```python
from build123d import *

# Parameters (mm, degrees)
SKETCH_1_R          = 3
SKETCH_1_R_2        = 5
EXTRUDE_1_DEPTH     = 4
CUT_EXTRUDE_1_DEPTH = 3


with BuildPart() as part:
    # 草图1 → 凸台-拉伸1 (new, symmetric)
    with BuildSketch(Plane(origin=(0, 0, 0), x_dir=(1, 0, 0), z_dir=(0, 1, 0))):
        with BuildLine():
            ThreePointArc((-0.330275229, 5.99090296), (-6, 0), (-0.330275229, -5.99090296))
            Line((-0.330275229, -5.99090296), (54.004587156, -8.98635444))
            ThreePointArc((54.004587156, -8.98635444), (63.5, 0), (54.004587156, 8.98635444))
            Line((54.004587156, 8.98635444), (-0.330275229, 5.99090296))
        make_face()
        with Locations(Location((0, 0, 0), (0, 0, 270))):
            Circle(SKETCH_1_R, mode=Mode.SUBTRACT)
        with Locations(Location((54.5, 0, 0), (0, 0, 270))):
            Circle(SKETCH_1_R_2, mode=Mode.SUBTRACT)
    extrude(amount=EXTRUDE_1_DEPTH, both=True)

    # 草图2 → 切除-拉伸1 (cut)
    with BuildSketch(Plane(origin=(0, 4, 0), x_dir=(1, 0, 0), z_dir=(0, 1, 0))):
        Polygon((26.837155963, 7.4886287), (11.750234203, -6.65689489), (-12.859516692, -6.65689489), (-12.859516692, 10.73344258), align=None)
    extrude(amount=-CUT_EXTRUDE_1_DEPTH, mode=Mode.SUBTRACT)


solid = part.part
```
Geometry check sheet. Reference: the model listing, model coordinates, mm. A direction names the side the tool comes from. Coordinates: 2 decimals unless noted, no trailing zeros. Loops run counter-clockwise (first coordinate to the right, second up) from the corner with the lowest first, then second, coordinate; pieces in that order, holes last. Notation, with made-up numbers: (-2.5, 62.25) -> (14.5, 62.25) arc R27 ccw to (14.5, 84.25) -> close; hole circle Ø11 at (37, 24.25). An arc over 180 degrees is marked (long way). Put each result on its own line as item: value.
1) Cross-section at B-B on y = -0.5. Record the boundary of the cut face in (x, z).
Result set:
outline: (-0.33, -5.99) -> (54, -8.99) arc R9 ccw (long way) to (54, 8.99) -> (-0.33, 5.99) arc R6 ccw to start; hole circle Ø6 at (0, 0); hole circle Ø10 at (54.5, 0)
2) Cross-section at D-D on z = 7.75. Record the boundary of the cut face in (x, y).
Result set:
outline: (31.58, -4) -> (59.08, -4) -> (59.08, 4) -> (31.58, 4) -> close
3) Release check for a two-part mould opening along Z. For faces 3 (the cylindrical face through (59.457, -0.056, -0.651)), 4 (the flat face through (26.457, 0.056, 7.468)), 5 (the flat face through (19.399, 2.521, -0.515)), 6 (the cylindrical face through (0.9, -1.54, 2.86)) record: released by +Z, released by -Z, zero draft, split by the parting line, or undercut.
Result set:
face 3: undercut
face 4: released by +Z
face 5: released by -Z
face 6: undercut
4) Cross-section at A-A on x = 58. Record the boundary of the cut face in (y, z).
Result set:
outline: (-4, -8.29) -> (4, -8.29) -> (4, -3.57) -> (-4, -3.57) -> close; (-4, 3.57) -> (4, 3.57) -> (4, 8.29) -> (-4, 8.29) -> close
5) Tool access check on faces 1 (the flat face through (7, 1, -1)), 2 (the flat face through (27.22, -0.83, -7.51)). Record the directions out of +Z, -Z, +X, -X, +Y, -Y that give a thin tool (end or side, any length) a straight path to the whole face; none if there is none.
Result set:
face 1: -Z, -X, +Y
face 2: -Z, -X, +Y, -Y
6) Gauge pin test, flat ends, axial feed: pin 1 Ø8 at (x, z) = (2.5, -3) entering from +Y; pin 2 Ø3 at (x, y) = (18.5, -2) entering from -Z; pin 3 Ø2 at (x, y) = (40, -2) entering from +Z. Record the tip position at first contact, or that the pin passes through.
Result set:
pin 1: stops at y = 1
pin 2: stops at z = -7.11
pin 3: stops at z = 8.27
7) Cross-section at C-C on z = 0. Record the boundary of the cut face in (x, y).
Result set:
outline: (-6, -4) -> (-3, -4) -> (-3, 1) -> (-6, 1) -> close; (3, -4) -> (49.5, -4) -> (49.5, 4) -> (18.85, 4) -> (18.85, 1) -> (3, 1) -> close; (59.5, -4) -> (63.5, -4) -> (63.5, 4) -> (59.5, 4) -> close
8) Thickness scan on line 1 (X direction, y = -2.5, z = -2.5); line 2 (X direction, y = -2.75, z = 1.25); line 3 (X direction, y = 3.75, z = 1.25). Record the ranges inside material, lowest first.
Result set:
line 1: x = -5.45 to -1.66, 1.66 to 50.17, 58.83 to 63.15
line 2: x = -5.87 to -2.73, 2.73 to 49.66, 59.34 to 63.41
line 3: x = 17.52 to 49.66, 59.34 to 63.41
